Answer from the drawing. Dimensions are ordinates in mm from the lowest x, y and z of the part. A direction names the side the tool comes from. Round coordinates to 2 decimals unless told otherwise and drop trailing zeros. Write each loop counter-clockwise with the first axis right and the second up, starting at its lowest first coordinate (ties: lowest second). Pieces come first, ordered by that corner, then holes.
1. Determine the mould class of the marked faces 3, 4 and 5 for opening direction X: pulls with the +X half, pulls with the -X half, needs draft (parallel to the pull), parting line crosses it, or undercut.
2. Find section C-C (z = 4.25). Write down the section's boundary in (x, y).
3. A tool of negligible diameter and unlimited length cuts with its end or side. For the marked faces 1 and 2, from which of +Z, -Z, +X, -X, +Y, -Y can it reach the whole face along a straight path? Write none if from no direction.
4. Find section D-D (x = 41.5). Write down the section's boundary in (y, z), and give its area (3 significant figures).
5. Find section B-B (z = 7.5). Write down the section's boundary in (x, y), and give its area (3 significant figures).
6. Straight lines are drawn through the part: probe 1 along X at (y, z) = (3.7, 7.5); probe 2 along X at (y, z) = (1.7, 13); probe 3 along Y at (x, z) = (13, 5.5). For each, find the intervals that lie inside material, in ascending order.
7. Find section A-A (x = 15). Write down the section's boundary in (y, z).
8. Flat-ended cylindrical pins translate along their axes: pin 1 Ø1.6 at (y, z) = (1, 11) entering from +X; pin 2 Ø8 at (x, z) = (12.5, 6.5) entering from -Y; pin 3 Ø1.5 at (y, z) = (2, 7) entering from +X; pin 4 Ø2 at (x, y) = (23.5, 2.5) entering from +Z. Find the tip coordinate at first contact, or state that the pin passes through.
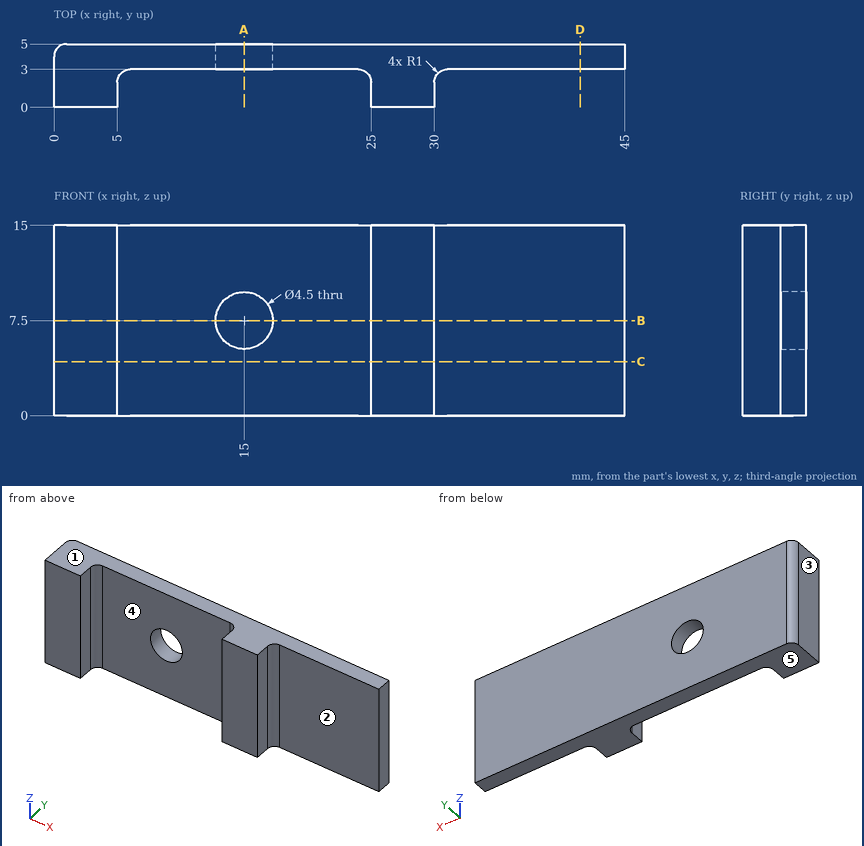
Worked answers:
1. face 3: pulls with the -X half
1. face 4: undercut
1. face 5: needs draft
2. outline: (0, 0) - (5, 0) - (5, 2) arc R1 cw to (6, 3) - (24, 3) arc R1 cw to (25, 2) - (25, 0) - (30, 0) - (30, 2) arc R1 cw to (31, 3) - (45, 3) - (45, 5) - (1, 5) arc R1 ccw to (0, 4) - close
3. face 1: +Z, +X, -X, +Y, -Y
3. face 2: +Z, -Z, +X, -Y
4. outline: (3, 0) - (5, 0) - (5, 15) - (3, 15) - close
4. area: 30.0 mm2
5. outline: (0, 0) - (5, 0) - (5, 2) arc R1 cw to (6, 3) - (12.75, 3) - (12.75, 5) - (1, 5) arc R1 ccw to (0, 4) - close; (17.25, 3) - (24, 3) arc R1 cw to (25, 2) - (25, 0) - (30, 0) - (30, 2) arc R1 cw to (31, 3) - (45, 3) - (45, 5) - (17.25, 5) - close
5. area: 111 mm2
6. probe 1: x = 0 to 12.75, 17.25 to 45
6. probe 2: x = 0 to 5, 25 to 30
6. probe 3: y = 3 to 5
7. outline: (3, 0) - (5, 0) - (5, 5.25) - (3, 5.25) - close; (3, 9.75) - (5, 9.75) - (5, 15) - (3, 15) - close
8. pin 1: stops at x = 30
8. pin 2: stops at y = 3
8. pin 3: stops at x = 30.34
8. pin 4: stops at z = 15
